Verification items for this drawing (mm, ordinates from the low corner). A direction names the side the tool comes from. Give positions to 0.01 mm unless a question says otherwise; leave off trailing zeros. Loops run counter-clockwise (first coordinate to the right, second up) from the corner with the lowest first, then second, coordinate; pieces in that order, holes last. Notation, with made-up numbers: M 58,-36.75 L 67,-36.75 A17 cw 67,-15.75 Z; hole C 14.25,71 d9. An arc over 180 degrees is marked long. Use a Markdown table: item, result.
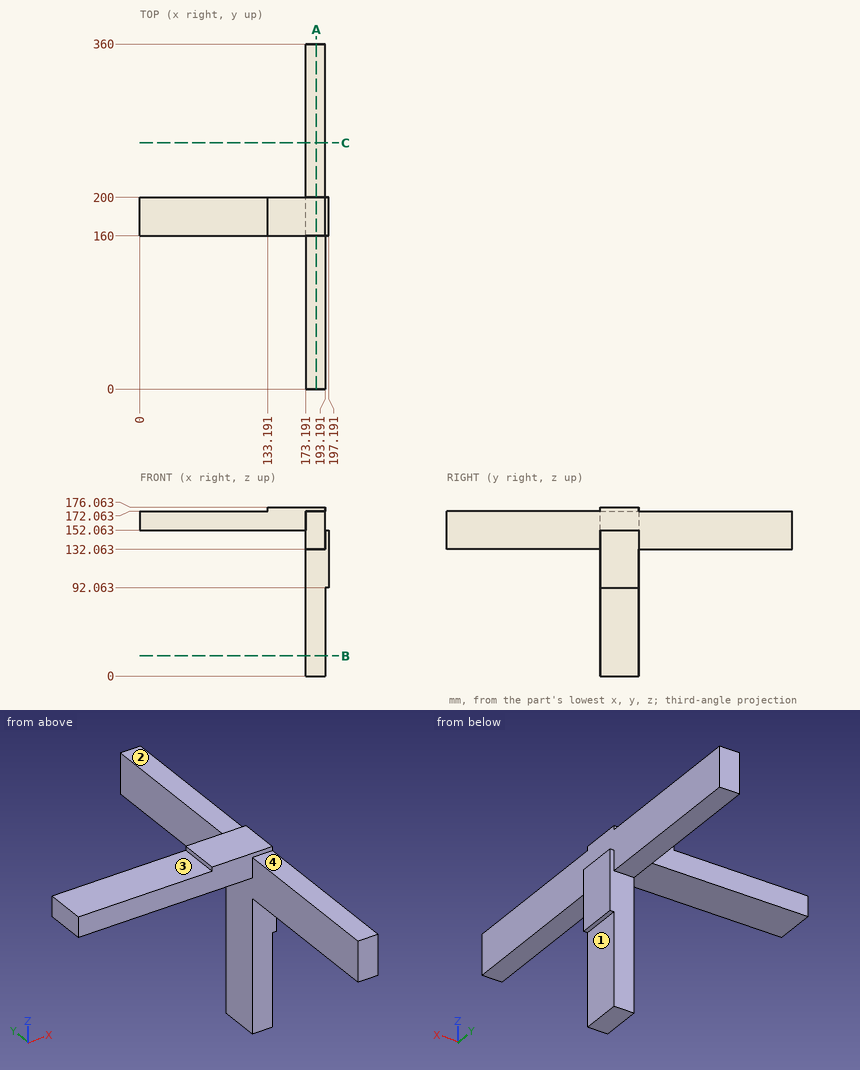
(1) Gauge pin test, flat ends, axial feed: P1, Ø2, axis at y = 172.5, z = 174, coming from the -X side; P2, Ø1.5, axis at y = 183.5, z = 85.5, coming from the -X side; P3, Ø7, axis at x = 187, z = 61.5, coming from the -Y side; P4, Ø12, axis at x = 43, y = 152, coming from the -Z side. Record the tip position at first contact, or that the pin passes through.
Results below:
| item | result |
|---|---|
| P1 | x = 133.19 |
| P2 | x = 173.19 |
| P3 | y = 160 |
| P4 | through |
(2) Cross-section at A-A on x = 184. Record the cut outline in (y, z), then the cut area to 3 significant figures.
Results below:
| item | result |
|---|---|
| outline | M 0,132.06 L 160,132.06 L 160,0 L 200,0 L 200,132.06 L 360,132.06 L 360,172.06 L 200,172.06 L 200,176.06 L 160,176.06 L 160,172.06 L 0,172.06 Z |
| area | 19,800 mm^2 |
(3) Cross-section at C-C on y = 257. Record the cut outline in (x, z).
Results below:
| item | result |
|---|---|
| outline | M 173.19,132.06 L 193.19,132.06 L 193.19,172.06 L 173.19,172.06 Z |
(4) Material ranges on line 1 (Y direction, x = 123, z = 158.5); line 2 (X direction, y = 318, z = 147); line 3 (X direction, y = 163.5, z = 101.5), recorded low to high.
Results below:
| item | result |
|---|---|
| line 1 | 160 to 200 |
| line 2 | 173.19 to 193.19 |
| line 3 | 173.19 to 197.19 |
(5) Set-up check for the marked faces 1, 2, 3 and 4: record each of +Z, -Z, +X, -X, +Y, -Y from which the full face is reachable in a straight line by a thin tool's end or side.
Results below:
| item | result |
|---|---|
| face 1 | -Z, +X, +Y, -Y |
| face 2 | +Z, +X, -X, +Y |
| face 3 | +Z, -X, +Y, -Y |
| face 4 | +Z, +X, -X, -Y |
(6) Cross-section at B-B on z = 21. Record the cut outline in (x, y), then the cut area to 3 significant figures.
Results below:
| item | result |
|---|---|
| outline | M 173.19,160 L 193.19,160 L 193.19,200 L 173.19,200 Z |
| area | 800 mm^2 |
